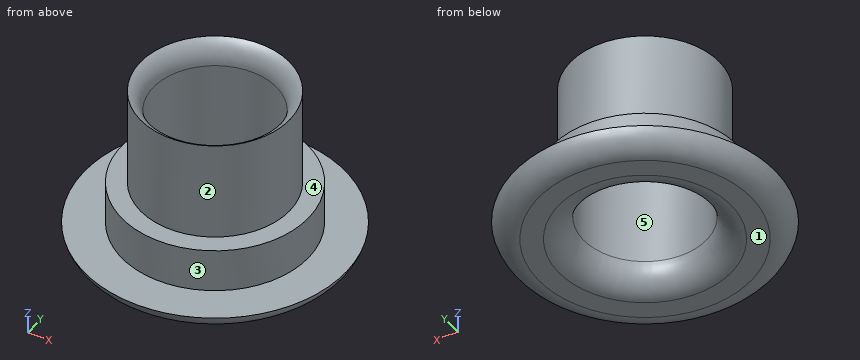
```python
from build123d import *

# Parameters (mm, degrees)
F0_R     = 10.5
F0_R_2   = 7.5
F1_DEPTH = 1.5
F0_R_3   = 4.95
F2_DEPTH = 13
F4_R     = 7.5
F4_R_2   = 6
F5_DEPTH = 8


# Not quite as in the source:
# - a fillet or chamfer that OpenCascade refuses, or shapes differently, is made with other operations: its cross-section is extruded or revolved along the edge and cut away or added
# - a feature names something its author has since deleted; it is built from what else it names


with BuildPart() as f1:
    # F0 (on Top) → F1 (new body)
    with BuildSketch(Plane.XY):
        Circle(F0_R)
        Circle(F0_R_2, mode=Mode.SUBTRACT)
    extrude(amount=F1_DEPTH)

    # F0 (on Top) → F2 (join)
    with BuildSketch(Plane.XY):
        Circle(F0_R_2)
        Circle(F0_R_3, mode=Mode.SUBTRACT)
    extrude(amount=F2_DEPTH)

    # F3: fillet of radius 2 on 1 edges, made by hand

    # F3_s1 → F3_t2 (revolve, cut)
    with BuildSketch(Plane.XZ):
        with BuildLine():
            ThreePointArc((10.5, 1.5), (9.7882531983, 0.4188611699), (8.5635083269, 0))
            Line((8.5635083269, 0), (10.5, 0))
            Line((10.5, 0), (10.5, 1.5))
        make_face()
    revolve(axis=Axis((0, 0, 0), (0, 0, 1)), mode=Mode.SUBTRACT)

    # F4 (on face) → F5 (cut)
    with BuildSketch(Plane.XY.offset(13)):
        Circle(F4_R)
        Circle(F4_R_2, mode=Mode.SUBTRACT)
    extrude(amount=-F5_DEPTH, mode=Mode.SUBTRACT)

    # F6: fillet of radius 2 on 2 edges, made by hand

    # F6_s1 → F6_t2 (revolve, cut)
    with BuildSketch(Plane.XZ):
        with BuildLine():
            ThreePointArc((6.95, 0), (5.5357864376, 0.5857864376), (4.95, 2))
            Line((4.95, 2), (4.95, 0))
            Line((4.95, 0), (6.95, 0))
        make_face()
    revolve(axis=Axis((0, 0, 0), (0, 0, 1)), mode=Mode.SUBTRACT)

    # F6_s3 → F6_t4 (revolve, cut)
    with BuildSketch(Plane.XZ):
        with BuildLine():
            ThreePointArc((4.95, 11.2400284093), (5.2324435963, 12.2647234859), (6, 13))
            Line((6, 13), (4.95, 13))
            Line((4.95, 13), (4.95, 11.2400284093))
        make_face()
    revolve(axis=Axis((0, 0, 13), (0, 0, 1)), mode=Mode.SUBTRACT)


solid = f1.part
```
Check sheet for the modelled part. Datum: model origin and axes. Units: mm. Face numbers are marked on the shaded views. A direction names the side the tool comes from. Give positions to 0.01 mm unless a question says otherwise; leave off trailing zeros. Loops run counter-clockwise (first coordinate to the right, second up) from the corner with the lowest first, then second, coordinate; pieces in that order, holes last. Notation, with made-up numbers: M 9,-27 L 51,-27 A19 ccw 51,-12 Z; hole C 39.5,44 d3. An arc over 180 degrees is marked long. Answer as CSV lines item,"result".
Item 1: Sectioned sample at C-C, the plane z = 3.75. Enter the section's corners in (x, y), then the cut area to 3 significant figures.
Reply:
outline,"C 0,0 d15; hole C 0,0 d9.9"
area,"99.7 mm^2"
Item 2: Draft check along X on the marked faces 3, 4 and 5. Enter one of: pulls with the +X half, pulls with the -X half, needs draft (parallel to the pull), parting line crosses it, or undercut.
Reply:
face 3,"parting line crosses it"
face 4,"needs draft"
face 5,"undercut"
Item 3: Sectioned sample at A-A, the plane y = 0. Enter the section's corners in (x, z).
Reply:
outline,"M -10.5,1.5 A2 ccw -8.56,0 L -6.95,0 A2 ccw -4.95,2 L -4.95,11.24 A2 ccw -6,13 L -6,5 L -7.5,5 L -7.5,1.5 Z; M 4.95,2 A2 ccw 6.95,0 L 8.56,0 A2 ccw 10.5,1.5 L 7.5,1.5 L 7.5,5 L 6,5 L 6,13 A2 ccw 4.95,11.24 Z"
Item 4: Depth check by flat-ended pin: pin 1 Ø5 at (x, y) = (1.5, -1) entering from -Z; pin 2 Ø1 at (y, z) = (-2, 7) entering from +X; pin 3 Ø1 at (x, z) = (-0.5, 7) entering from +Y; pin 4 Ø5 at (x, z) = (4, 10) entering from -Y. Enter the tip coordinate at first touch or a pass-through.
Reply:
pin 1,"through"
pin 2,"x = 5.81"
pin 3,"y = 6"
pin 4,"y = -5.81"
Item 5: Scan lines: L1, parallel to Y at x = 0, z = 9.25; L2, parallel to Y at x = 0, z = 4; L3, parallel to Z at x = 6.25, y = 5. Record each from-to range of solid material in increasing order.
Reply:
L1,"-6 to -4.95, 4.95 to 6"
L2,"-7.5 to -4.95, 4.95 to 7.5"
L3,"0 to 1.5"
Item 6: Set-up check for the marked faces 1 and 2: record each of +Z, -Z, +X, -X, +Y, -Y from which the full face is reachable in a straight line by a thin tool's end or side.
Reply:
face 1,"-Z, +X, -X, +Y, -Y"
face 2,"+Z"
Item 7: Sectioned sample at D-D, the plane z = 5.75. Enter the section's corners in (x, y), then the cut area to 3 significant figures.
Reply:
outline,"C 0,0 d12; hole C 0,0 d9.9"
area,"36.1 mm^2"
